Geometry check sheet. Reference: the model listing, model coordinates, mm. A direction names the side the tool comes from. Give positions to 0.01 mm unless a question says otherwise; leave off trailing zeros. Loops run counter-clockwise (first coordinate to the right, second up) from the corner with the lowest first, then second, coordinate; pieces in that order, holes last. Notation, with made-up numbers: (-12, 21) -> (46, 21) arc R23 cw to (46, 57) -> close; hole circle Ø5 at (33, 13). An arc over 180 degrees is marked (long way). Write item = value, one per line.
```python
from build123d import *

# Parameters (mm, degrees)
F0_R      = 63.5
F0_R_2    = 16.637
F1_DEPTH  = 66.675
F2_R      = 63.5
F2_R_2    = 8.73125
F3_DEPTH  = 66.676
F4_R      = 8.73125
F5_DEPTH  = 19.05
F7_R      = 15.1150654982
F8_DEPTH  = 53.594
F9_R      = 3.175
F10_DEPTH = 25.4


# Not quite as in the source:
# - a pattern or mirror of a feature is missing from the dataset's text; its kind, count and spacing are read off the source's solid


with BuildPart() as f1:
    # F0 (on Front) → F1 (new body)
    with BuildSketch(Plane.XZ):
        Circle(F0_R)
        Circle(F0_R_2, mode=Mode.SUBTRACT)
    extrude(amount=F1_DEPTH)

    # F2 (on face) → F3 (cut, through all)
    with BuildSketch(Plane.XZ.offset(66.675)):
        Circle(F2_R)
        with BuildLine():
            Line((-31.75, 0), (-31.75, 53.975))
            Line((-31.75, 53.975), (31.7028198831, 53.975))
            ThreePointArc((31.7028198831, 53.975), (38.3398958316, 34.3431316591), (51.2105212065, 18.1009632644))
            ThreePointArc((51.2105212065, 18.1009632644), (52.3246389461, 17.2136710516), (53.5311013852, 16.4567072537))
            ThreePointArc((53.5311013852, 16.4567072537), (62.6217032006, -4.8040419219), (44.2117641598, -18.7944901416))
            Line((44.2117641598, -18.7944901416), (31.3671737764, -18.7944901416))
            ThreePointArc((31.3671737764, -18.7944901416), (26.5189786011, -19.756304441), (22.405124126, -22.4960643869))
            ThreePointArc((22.405124126, -22.4960643869), (-12.179897557, -29.3208559817), (-31.75, 0))
        make_face(mode=Mode.SUBTRACT)
        with Locations((44.45, 0)):
            Circle(F2_R_2)
    extrude(amount=-F3_DEPTH, mode=Mode.SUBTRACT)

    # F4 (on face) → F5 (cut)
    with BuildSketch(Plane.XZ.offset(66.675)):
        with BuildLine():
            Line((31.3671737764, -18.7944901416), (44.2117641598, -18.7944901416))
            ThreePointArc((44.2117641598, -18.7944901416), (62.6217032006, -4.8040419219), (53.5311013852, 16.4567072537))
            ThreePointArc((53.5311013852, 16.4567072537), (52.3246389461, 17.2136710516), (51.2105212065, 18.1009632644))
            ThreePointArc((51.2105212065, 18.1009632644), (38.3398958316, 34.3431316591), (31.7028198831, 53.975))
            Line((31.7028198831, 53.975), (31.7499514816, 0.0555059775))
            ThreePointArc((31.7499514816, 0.0555059775), (31.7499878704, 0.0277529994), (31.75, 0))
            ThreePointArc((31.75, 0), (29.3208559817, -12.179897557), (22.405124126, -22.4960643869))
            ThreePointArc((22.405124126, -22.4960643869), (26.5189786011, -19.756304441), (31.3671737764, -18.7944901416))
        make_face()
        with Locations((44.45, 0)):
            Circle(F4_R, mode=Mode.SUBTRACT)
    f5 = extrude(amount=-F5_DEPTH, mode=Mode.SUBTRACT)

    # F5_copies: F5 across plane
    add(f5.mirror(Plane.ZX.offset(-33.3375)), mode=Mode.SUBTRACT)

    # F7 (on face) → F8 (cut)
    with BuildSketch(Plane.XY.offset(53.975)):
        with Locations((0, -33.3375)):
            Circle(F7_R)
    extrude(amount=-F8_DEPTH, mode=Mode.SUBTRACT)

    # F9 (on face) → F10 (cut)
    with BuildSketch(Plane(origin=(0, 0, 0), x_dir=(-1, 0, 0), z_dir=(0, 1, 0))):
        with Locations((0, 42.8625)):
            Circle(F9_R)
    extrude(amount=-F10_DEPTH, mode=Mode.SUBTRACT)


solid = f1.part
```
Item 1: Gauge pin test, flat ends, axial feed: pin 1 (10 mm diameter, centred on y = -17, z = 17.5, fed in from +X); pin 2 (6.5 mm diameter, centred on x = 40.5, y = -27.5, fed in from -Z); pin 3 (1.5 mm diameter, centred on x = 22.5, z = 4.5, fed in from +Y); pin 4 (24 mm diameter, centred on x = 0, y = -33.34, fed in from +Z). Record the tip position at first contact, or that the pin passes through.
Answer:
pin_1 = 58.08
pin_2 = -18.79
pin_3 = 0
pin_4 = -11.52
Item 2: Tool access check on faces 5 (the cylindrical face through (13.96, -39.13, 30.79)), 6 (the cylindrical face through (38.2, -33.5, 34.6)), 7 (the cylindrical face through (0.41, -9.15, 46.01)), 8 (the flat face through (38, -34, -18.794)). Record the directions out of +Z, -Z, +X, -X, +Y, -Y that give a thin tool (end or side, any length) a straight path to the whole face; none if there is none.
Answer:
face_5 = +Z
face_6 = +Z, +X, +Y, -Y
face_7 = +Y
face_8 = -Z, +X, +Y, -Y
Item 3: Draft check along Z on faces 1 (the cylindrical face through (35.727, -33.538, 0.384)), 2 (the flat face through (38, -19.05, 8)), 3 (the cylindrical face through (-3.61, -32.87, -16.24)), 4 (the cylindrical face through (62.7, -33.5, -4.5)). Enter one of: +Z half, -Z half, draft (parallel to the pull), parting line (faces both ways), or undercut.
Answer:
face_1 = undercut
face_2 = draft
face_3 = undercut
face_4 = parting line
Item 4: Section check A-A, the plane x = 0. Give the number of separate pieces and of enclosed holes in the cut face, plus the area to 3 significant figures.
Answer:
separate_pieces = 4
enclosed_holes = 0
area = 2,250 mm^2
Item 5: Thickness scan on L1, parallel to X at y = -14, z = 24; L2, parallel to Y at x = 33, z = -1.5 (3 decimals); L3, parallel to Z at x = -14.5, y = -12 (3 decimals). Record the ranges inside material, lowest first. Write a range as [from, to].
Answer:
L1 = [-31.75, 31.73]
L2 = [-47.625, -19.05]
L3 = [-28.246, -8.157], [8.157, 53.975]
Item 6: Section check B-B, the plane z = -14. Record the cut outline in (x, y) (3 decimals), plus the area to 3 significant figures.
Answer:
outline = (-28.497, -66.675) -> (-8.988, -66.675) -> (-8.988, 0) -> (-28.497, 0) -> close; (8.988, -66.675) -> (28.497, -66.675) -> (28.497, -47.625) -> (56.992, -47.625) -> (56.992, -19.05) -> (28.497, -19.05) -> (28.497, 0) -> (8.988, 0) -> close
area = 3,420 mm^2
